Study the drawing (mm; zero at the part's minimum x, y, z) and answer. A direction names the side the tool comes from. Coordinates: 2 decimals unless noted, no trailing zeros. Order: outer loops, then holes, each group sorted by start corner. A loop starts at its lowest first (then second) coordinate and runs counter-clockwise, first axis right, second up. Notation, with made-up numbers: M 82.25,-34.5 L 115.25,-34.5 A13 ccw 115.25,-17.5 Z; hole C -28,10 d2. An arc over 180 degrees is marked long. Use a Markdown table: item, result. Add a question column.
1) Find section D-D on y = 37. Write down the section's boundary in (x, z), plus the area to 3 significant figures.
2) The mould has two halves that part along X. Classify the marked faces 4, 5 and 6: released by +X, released by -X, zero draft, split by the parting line, or undercut.
3) Find section A-A on z = 10. Write down the section's boundary in (x, y), plus the area to 3 significant figures.
4) Find the intervals of material crossed by probe 1 along Z at (x, y) = (7.5, 2.85); probe 2 along X at (y, z) = (1.1, 10); probe 3 along X at (y, z) = (25, 10), in increasing order. Write a range as [from, to].
5) Find section B-B on z = 30.9. Write down the section's boundary in (x, y), plus the area to 3 significant figures.
6) Find section C-C on x = 68.5. Write down the section's boundary in (y, z).
7) For the marked faces 1, 2 and 3, determine the directions among +Z, -Z, +X, -X, +Y, -Y from which every point of the face is accessible in a straight line to the end or side of a thin tool.
8) Each of these flat-tipped pins is pushed along its axis until it touches: pin 1 Ø12 at (x, y) = (45, 34.5) entering from +Z; pin 2 Ø10 at (y, z) = (10.5, 20.5) entering from +X (3 decimals); pin 3 Ø2 at (x, z) = (7.5, 10) entering from +Y; pin 4 Ø1 at (y, z) = (14.5, 19) entering from -X. Where does it stop, or does it pass through?
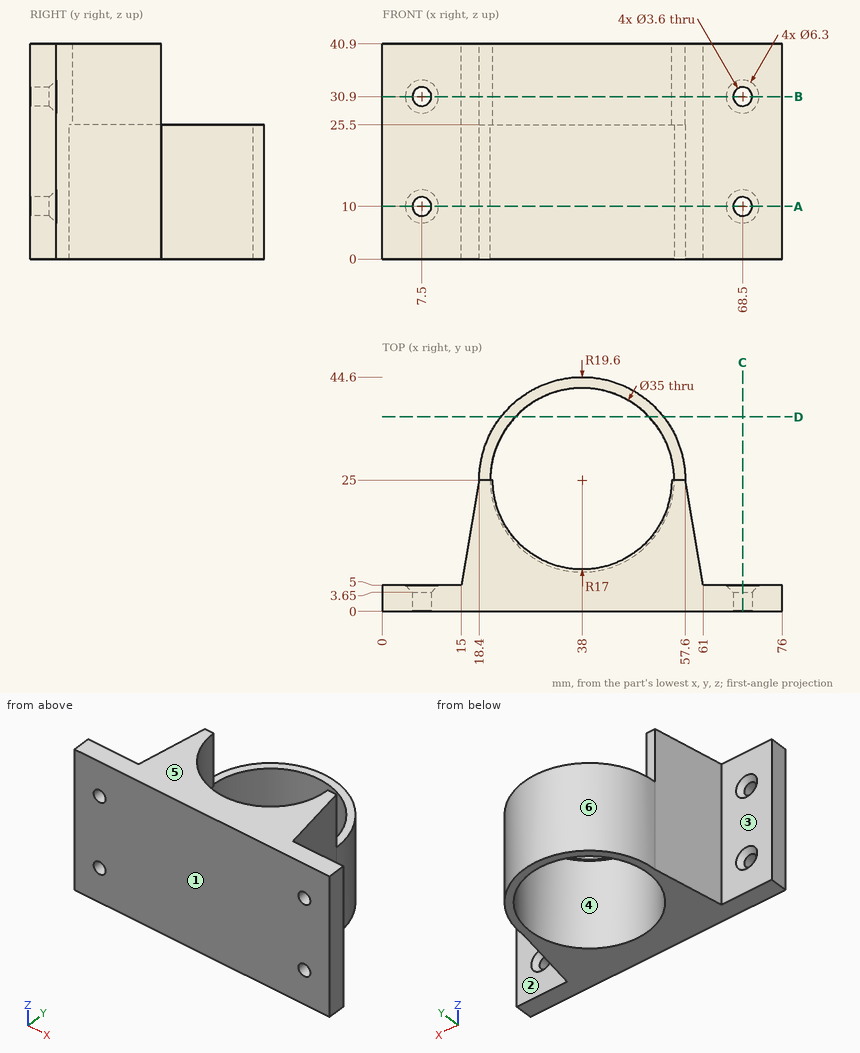
Check result:
| question | item | result |
|---|---|---|
| 1 | outline | M 22.5,0 L 25.26,0 L 25.26,25.5 L 22.5,25.5 Z; M 50.74,0 L 53.5,0 L 53.5,25.5 L 50.74,25.5 Z |
| 1 | area | 141 mm2 |
| 2 | face 4 | undercut |
| 2 | face 5 | zero draft |
| 2 | face 6 | split by the parting line |
| 3 | outline | M 0,0 L 5.7,0 L 5.7,3.65 L 4.35,5 L 0,5 Z; M 9.3,0 L 66.7,0 L 66.7,3.65 L 65.35,5 L 61,5 L 57.6,25 A19.6 ccw 18.4,25 L 15,5 L 10.65,5 L 9.3,3.65 Z; M 70.3,0 L 76,0 L 76,5 L 71.65,5 L 70.3,3.65 Z; hole C 38,25 d35 |
| 3 | area | 834 mm2 |
| 4 | probe 1 | z = [0, 8.2], [11.8, 29.1], [32.7, 40.9] |
| 4 | probe 2 | x = [0, 5.7], [9.3, 66.7], [70.3, 76] |
| 4 | probe 3 | x = [18.4, 20.5], [55.5, 57.6] |
| 5 | outline | M 0,0 L 5.7,0 L 5.7,3.65 L 4.35,5 L 0,5 Z; M 9.3,0 L 66.7,0 L 66.7,3.65 L 65.35,5 L 61,5 L 57.6,25 L 55,25 A17 cw 21,25 L 18.4,25 L 15,5 L 10.65,5 L 9.3,3.65 Z; M 70.3,0 L 76,0 L 76,5 L 71.65,5 L 70.3,3.65 Z |
| 5 | area | 738 mm2 |
| 6 | outline | M 0,0 L 5,0 L 5,6.85 L 3.65,8.2 L 0,8.2 Z; M 0,11.8 L 3.65,11.8 L 5,13.15 L 5,27.75 L 3.65,29.1 L 0,29.1 Z; M 0,32.7 L 3.65,32.7 L 5,34.05 L 5,40.9 L 0,40.9 Z |
| 7 | face 1 | +Z, -Z, +X, -X, -Y |
| 7 | face 2 | +Z, -Z, +X, +Y |
| 7 | face 3 | +Z, -Z, -X, +Y |
| 8 | pin 1 | stops at z = 25.5 |
| 8 | pin 2 | stops at x = 60.915 |
| 8 | pin 3 | passes through |
| 8 | pin 4 | stops at x = 16.53 |
